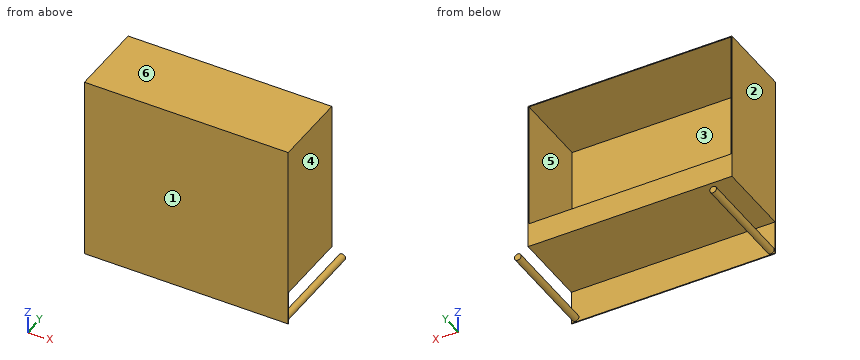
Autodesk Inventor part; units mm, degrees
ref_plane "YZ Plane" through (0, 0, 0) normal (1, 0, 0) x (0, 1, 0)
ref_plane "XZ Plane" through (0, 0, 0) normal (0, 1, 0) x (-1, 0, 0)
ref_plane "XY Plane" through (0, 0, 0) normal (0, 0, 1) x (1, 0, 0)
sketch "Sketch1" plane through (0, 0, 0) normal (0, 1, 0) x (-1, 0, 0)
  line L0 (-600, 450) -> (600, 450)
  line L1 (600, 450) -> (600, -450)
  line L2 (600, -450) -> (-600, -450)
  line L3 (-600, -450) -> (-600, 450)
  line L4 (-600, 450) -> (600, -450) construction
  line L5 (600, 450) -> (-600, -450) construction
  line L6 (595, 445) -> (-595, 445)
  line L7 (-595, 445) -> (-595, -305)
  line L8 (-595, -305) -> (595, -305)
  line L9 (595, -305) -> (595, 445)
  point P0 (0, 0)
  dimension "d0" = 1200
  dimension "d1" = 900
  dimension "d2" = 1190
  dimension "d3" = 750
extrude "Extrusion1" add sketch "Sketch1" along normal blind 450
ref_plane "Work Plane3" through (0, 0, 0) normal (0, 1, 0) x (1, 0, 0)
sketch "Sketch4" plane through (0, 0, 0) normal (0, 1, 0) x (1, 0, 0)
  line L0 (600, 450) -> (-600, 450)
  line L1 (-600, 450) -> (600, 450)
  line L2 (600, 450) -> (600, 650)
  line L3 (600, 650) -> (-600, 650)
  line L4 (-600, 650) -> (-600, 450)
  circle A0 centre (-575, 625) radius 20
  circle A1 centre (575, 625) radius 20
  point P0 (0, 0)
  dimension "d12" = 1200
  dimension "d13" = 200
  dimension "d14" = 40
  dimension "d15" = 40
extrude "Extrusion2" add sketch "Sketch4" along normal blind 600 contours A0 | A1
ref_plane "Work Plane6" through (0, 0, 0) normal (0, 1, 0) x (1, 0, 0)
sketch "Sketch5" plane through (0, 0, 0) normal (0, 1, 0) x (1, 0, 0)
  line L0 (-600, 450) -> (600, 450)
  line L1 (600, 450) -> (600, 650)
  line L2 (600, 650) -> (-600, 650)
  line L3 (-600, 650) -> (-600, 450)
  point P0 (0, 0)
  dimension "d18" = 1200
  dimension "d19" = 200
extrude "Extrusion3" add sketch "Sketch5" along normal blind 5
ref_plane "Work Plane7" through (0, 0, 0) normal (0, 1, 0) x (1, 0, 0)
sketch "Sketch6" plane through (0, 0, 0) normal (0, 1, 0) x (1, 0, 0)
  line L0 (-595, 305) -> (595, 305)
  line L1 (595, -445) -> (-595, -445)
  line L2 (595, 305) -> (-595, 305)
  line L3 (-595, 305) -> (-595, -445)
  line L4 (-595, -445) -> (595, -445)
  line L5 (595, -445) -> (595, 305)
  point P0 (0, 0)
extrude "Extrusion4" add sketch "Sketch6" along normal blind 5
properties part number "Distanced Top Bin"
Here's how the part is built. I have some questions about the finished solid (model axes, mm). Face numbers are marked on the shaded views. A direction names the side the tool comes from. Give positions to 0.01 mm unless a question says otherwise; leave off trailing zeros. Loops run counter-clockwise (first coordinate to the right, second up) from the corner with the lowest first, then second, coordinate; pieces in that order, holes last. Notation, with made-up numbers: (-5.5, -7.75) -> (6.5, -7.75) arc R21 ccw to (6.5, 19.25) -> close; hole circle Ø7 at (59.5, 75). An arc over 180 degrees is marked (long way). Use one line per item in the form item = value. Start each with the question number.
1) Please list where these lines run through material, in increasing order: line 1 along Z through (x, y) = (143, 323); line 2 along X through (y, z) = (125, -233.5); line 3 along Y through (x, z) = (508, -375.5).
2) For P1, Ø1, axis at x = 245, z = 280, coming from the -Y side; P2, Ø3, axis at x = -302, z = -173, coming from the +Y side, each with a flat end and sliding along its axis, tell me the tip position at first contact or that it passes through.
3) Thinking about a two-plate mould opening in X: for the marked faces 1, 2, 3 and 4, which applies, +X half, -X half, draft (parallel to the pull), parting line (faces both ways), or undercut?
4) Imagine slicing it at A-A (y = 252.5). Please give me the cut outline in (x, z).
5) Imagine slicing it at B-B (x = -575). Please give me the cut outline in (y, z), then the cut area to 4 significant figures.
6) Which directions (+Z, -Z, +X, -X, +Y, -Y) give clear straight access to the entire face, cutting with the end or side of a thin tool? Please do the marked faces 5 and 6.
7) Imagine slicing it at D-D (x = 107). Please give me the cut outline in (y, z), then the cut area to 4 significant figures.
8) Imagine slicing it at C-C (z = 169). Please give me the cut outline in (x, y).
Check values:
q1.line_1 = -450 to -305, 445 to 450
q1.line_2 = -600 to -595, 595 to 600
q1.line_3 = 0 to 450
q2.P1 = 0
q2.P2 = 5
q3.face_1 = draft
q3.face_2 = -X half
q3.face_3 = undercut
q3.face_4 = +X half
q4.outline = (-600, -450) -> (600, -450) -> (600, 450) -> (-600, 450) -> close; circle Ø40 at (-575, -625); circle Ø40 at (575, -625); hole (-595, -305) -> (595, -305) -> (595, 445) -> (-595, 445) -> close
q5.outline = (0, -650) -> (5, -650) -> (5, -645) -> (600, -645) -> (600, -605) -> (5, -605) -> (5, -450) -> (450, -450) -> (450, -305) -> (5, -305) -> (5, 445) -> (450, 445) -> (450, 450) -> (0, 450) -> close
q5.area = 96,050 mm^2
q6.face_5 = +Y
q6.face_6 = +Z, +X, -X, +Y, -Y
q7.outline = (0, -650) -> (5, -650) -> (5, -450) -> (450, -450) -> (450, -305) -> (5, -305) -> (5, 445) -> (450, 445) -> (450, 450) -> (0, 450) -> close
q7.area = 72,250 mm^2
q8.outline = (-600, 0) -> (600, 0) -> (600, 450) -> (595, 450) -> (595, 5) -> (-595, 5) -> (-595, 450) -> (-600, 450) -> close
